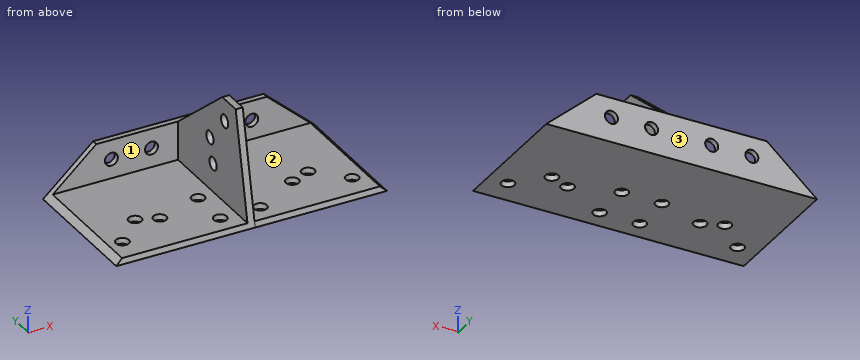
```python
from build123d import *

# Parameters (mm, degrees)
SKETCH_1_W          = 540
SKETCH_1_H          = 265
SKETCH_1_R          = 13
EXTRUDE_548_DEPTH   = 11.5
SKETCH_2_W          = 540
SKETCH_2_H          = 11.5
EXTRUDE_1_DEPTH     = 77.5
CUT_EXTRUDE_1_DEPTH = 609.067430471
SKETCH_4_R          = 13
CUT_EXTRUDE_2_DEPTH = 609.067430471
SKETCH_5_W          = 14
SKETCH_5_H          = 253.5
EXTRUDE_2_DEPTH     = 208.5
SKETCH_6_R          = 13
CUT_EXTRUDE_3_DEPTH = 442.988687638
CUT_EXTRUDE_4_DEPTH = 442.988687638


with BuildPart() as part:
    # 草图1 → Extrude 548 (new body)
    with BuildSketch(Plane.XY):
        with Locations((270, 132.5)):
            Rectangle(SKETCH_1_W, SKETCH_1_H)
        with Locations((97.46594539, 108.46594539)):
            Circle(SKETCH_1_R, mode=Mode.SUBTRACT)
        with Locations((40.897402896, 51.897402896)):
            Circle(SKETCH_1_R, mode=Mode.SUBTRACT)
        with Locations(Location((499.102597104, 51.897402896, 0), (0, 0, 180))):
            Circle(SKETCH_1_R, mode=Mode.SUBTRACT)
        with Locations(Location((402.170987639, 92.261534081, 0), (0, 0, 180))):
            Circle(SKETCH_1_R, mode=Mode.SUBTRACT)
        with Locations((230, 121)):
            Circle(SKETCH_1_R, mode=Mode.SUBTRACT)
        with Locations((230, 41)):
            Circle(SKETCH_1_R, mode=Mode.SUBTRACT)
        with Locations(Location((310, 41, 0), (0, 0, 180))):
            Circle(SKETCH_1_R, mode=Mode.SUBTRACT)
        with Locations(Location((310, 121, 0), (0, 0, 180))):
            Circle(SKETCH_1_R, mode=Mode.SUBTRACT)
        with Locations((137.829012361, 92.261534081)):
            Circle(SKETCH_1_R, mode=Mode.SUBTRACT)
        with Locations(Location((442.53405461, 108.46594539, 0), (0, 0, 180))):
            Circle(SKETCH_1_R, mode=Mode.SUBTRACT)
    extrude(amount=EXTRUDE_548_DEPTH)

    # 草图2 → 凸台-拉伸1 (add)
    with BuildSketch(Plane.XY.offset(11.5)):
        with Locations((270, 259.25)):
            Rectangle(SKETCH_2_W, SKETCH_2_H)
    extrude(amount=EXTRUDE_1_DEPTH)

    # 草图3 → 切除-拉伸1 (cut, through all)
    with BuildSketch(Plane(origin=(0, 265, 0), x_dir=(-1, 0, 0), z_dir=(0, 1, 0))):
        Polygon((0, 0), (-100, 89), (0, 89), align=None)
        Polygon((-540, 0), (-440, 89), (-540, 89), align=None)
    extrude(amount=-CUT_EXTRUDE_1_DEPTH, mode=Mode.SUBTRACT)

    # 草图4 → 切除-拉伸2 (cut, through all)
    with BuildSketch(Plane(origin=(0, 265, 0), x_dir=(-1, 0, 0), z_dir=(0, 1, 0))):
        with Locations(Location((-210, 50, 0), (0, 0, 90))):
            Circle(SKETCH_4_R)
        with Locations(Location((-130, 50, 0), (0, 0, 90))):
            Circle(SKETCH_4_R)
        with Locations(Location((-410, 50, 0), (0, 0, 90))):
            Circle(SKETCH_4_R)
        with Locations(Location((-330, 50, 0), (0, 0, 90))):
            Circle(SKETCH_4_R)
    extrude(amount=-CUT_EXTRUDE_2_DEPTH, mode=Mode.SUBTRACT)

    # 草图5 → 凸台-拉伸2 (add)
    with BuildSketch(Plane.XY.offset(11.5)):
        with Locations((270, 126.75)):
            Rectangle(SKETCH_5_W, SKETCH_5_H)
    extrude(amount=EXTRUDE_2_DEPTH)

    # 草图6 → 切除-拉伸3 (cut, through all)
    with BuildSketch(Plane(origin=(277, 0, 0), x_dir=(0, 0, -1), z_dir=(1, 0, 0))):
        with Locations((-115.693003517, 138.161774652)):
            Circle(SKETCH_6_R)
        with Locations((-175.485749012, 85.012667545)):
            Circle(SKETCH_6_R)
        with Locations((-68.400421337, 126.93798921)):
            Circle(SKETCH_6_R)
        Polygon((-89, 253.5), (-220, 93.5), (-220, 253.5), align=None)
        Polygon((-220, 45), (0, 0), (-220, 0), align=None)
    extrude(amount=-CUT_EXTRUDE_3_DEPTH, mode=Mode.SUBTRACT)

    # 草图7 → 切除-拉伸4 (cut, through all)
    with BuildSketch(Plane.ZY.offset(-277)):
        Polygon((0, 0), (11.5, 2.352272727), (11.5, 0), align=None)
    extrude(amount=-CUT_EXTRUDE_4_DEPTH, mode=Mode.SUBTRACT)


solid = part.part
```
CAD build for the part. Positions are in the model's coordinates, mm. Face numbers are marked on the shaded views. A direction names the side the tool comes from. Coordinates: 2 decimals unless noted, no trailing zeros. Order: outer loops, then holes, each group sorted by start corner. A loop starts at its lowest first (then second) coordinate and runs counter-clockwise, first axis right, second up. Notation, with made-up numbers: (48, 76.5) - (81, 76.5) arc R17 cw to (81, 97.5) - close; hole circle Ø3 at (37, 1.5). An arc over 180 degrees is marked (long way). Answer in a Markdown table with one row per item.
1. Drill centre lines: L1, parallel to Y at x = 310, z = 7; L2, parallel to Y at x = 230, z = 7.25; L3, parallel to Z at x = 35, y = 98. Where is each one in solid material? Low to high. Write a range as from..to.
Answer:
| item | result |
|---|---|
| L1 | 1.43..28, 54..108, 134..265 |
| L2 | 1.48..28, 54..108, 134..265 |
| L3 | 0..11.5 |
2. Slice it at B-B, the plane z = 112. List the corners of the cut face in (x, y).
Answer:
| item | result |
|---|---|
| outline | (263, 22.91) - (277, 22.91) - (277, 125.7) - (263, 125.7) - close; (263, 150.63) - (277, 150.63) - (277, 225.41) - (263, 225.41) - close |
3. 3-axis set-ups, long thin cutter, end or side, ignore diameter. For the marked faces 1, 2 and 3: which of +Z, -Z, +X, -X, +Y, -Y reach the whole face in a straight line?
Answer:
| item | result |
|---|---|
| face 1 | +Z, -X, -Y |
| face 2 | +Z, +X, -Y |
| face 3 | +Z, -Z, +X, -X, +Y |
4. Slice it at C-C, the plane x = 230. List the corners of the cut face in (y, z), then the cut area to 3 significant figures.
Answer:
| item | result |
|---|---|
| outline | (0, 0) - (28, 0) - (28, 11.5) - (2.35, 11.5) - close; (54, 0) - (108, 0) - (108, 11.5) - (54, 11.5) - close; (134, 0) - (265, 0) - (265, 89) - (253.5, 89) - (253.5, 11.5) - (134, 11.5) - close |
| area | 3,330 mm² |
5. Flat gauge pins, fed straight in: P1, Ø8, axis at y = 166.5, z = 114.5, coming from the -X side; P2, Ø4, axis at x = 288, y = 161, coming from the +Z side; P3, Ø12, axis at x = 279, z = 137, coming from the +Y side. Where does each tip first touch, or does it go through?
Answer:
| item | result |
|---|---|
| P1 | x = 263 |
| P2 | z = 11.5 |
| P3 | y = 201.78 |
6. Slice it at D-D, the plane y = 219.5. List the corners of the cut face in (x, z), then the cut area to 3 significant figures.
Answer:
| item | result |
|---|---|
| outline | (0, 0) - (540, 0) - (527.08, 11.5) - (277, 11.5) - (277, 116.84) - (263, 116.84) - (263, 11.5) - (12.92, 11.5) - close |
| area | 7,540 mm² |
7. Slice it at A-A, the plane x = 330. List the corners of the cut face in (y, z).
Answer:
| item | result |
|---|---|
| outline | (0, 0) - (265, 0) - (265, 37) - (253.5, 37) - (253.5, 11.5) - (2.35, 11.5) - close; (253.5, 63) - (265, 63) - (265, 89) - (253.5, 89) - close |
